Geometry check sheet. Reference: the model listing, model coordinates, mm. A direction names the side the tool comes from. Give positions to 0.01 mm unless a question says otherwise; leave off trailing zeros. Write each loop counter-clockwise with the first axis right and the second up, starting at its lowest first coordinate (ties: lowest second). Pieces come first, ordered by that corner, then holes. Notation, with made-up numbers: (-15, 15) -> (6, 15) arc R32 cw to (6, 49) -> close; hole circle Ø5 at (75, -20). An arc over 180 degrees is marked (long way). Use a Markdown table: item, result. Add a question column.
Autodesk Inventor part; units mm, degrees
ref_plane "YZ Plane" through (0, 0, 0) normal (1, 0, 0) x (0, 1, 0)
ref_plane "XZ Plane" through (0, 0, 0) normal (0, 1, 0) x (-1, 0, 0)
ref_plane "XY Plane" through (0, 0, 0) normal (0, 0, 1) x (1, 0, 0)
sketch "Эскиз1" plane through (0, 0, 0) normal (0, 1, 0) x (-1, 0, 0)
  line L0 (-155, 270) -> (155, 270)
  line L1 (155, 270) -> (155, -270)
  line L2 (155, -270) -> (-155, -270)
  line L3 (-155, -270) -> (-155, 270)
  line L4 (-155, 270) -> (155, -270) construction
  line L5 (155, 270) -> (-155, -270) construction
  circle A0 centre (0, 0) radius 50
  dimension "d0" = 310
  dimension "d1" = 540
  dimension "d2" = 100
extrude "Выдавливание1" add sketch "Эскиз1" along normal blind 4
sketch "Эскиз2" plane through (0, 4, 0) normal (0, 1, 0) x (1, 0, 0)
  line L0 (153, 268) -> (-153, 268)
  line L1 (-153, 268) -> (-153, -268)
  line L2 (-153, -268) -> (153, -268)
  line L3 (153, -268) -> (153, 268)
  line L4 (153, 268) -> (-153, -268) construction
  line L5 (-153, 268) -> (153, -268) construction
  line L6 (-155, 270) -> (-155, -270)
  line L7 (155, 270) -> (-155, 270)
  line L8 (-155, 270) -> (-155, -270)
  line L9 (-155, -270) -> (155, -270)
  line L10 (155, -270) -> (155, 270)
  line L11 (155, 270) -> (-155, -270) construction
  line L12 (-155, 270) -> (155, -270) construction
  point P0 (0, 0)
  dimension "d5" = 306
  dimension "d6" = 536
extrude "Выдавливание2" add sketch "Эскиз2" along normal blind 40
sketch "Эскиз3" plane through (0, 4, 0) normal (0, 1, 0) x (1, 0, 0)
  circle A0 centre (0, 0) radius 50
  circle A1 centre (0, 0) radius 60
  dimension "d9" = 120
extrude "Выдавливание3" add sketch "Эскиз3" along normal blind 40
properties part number "ЗЕМЛЯЕМКОСТЬ"
1) Sectioned sample at D-D, the plane x = -110. Enter the section's corners in (y, z), and give its area (3 significant figures).
2) Sectioned sample at B-B, the plane z = 0. Enter the section's corners in (x, y), and give its area (3 significant figures).
3) Material ranges on probe 1 along Z at (x, y) = (0, 31); probe 2 along X at (y, z) = (23.5, 0); probe 3 along X at (y, z) = (35, -207), recorded low to high. Write a range as [from, to].
4) Gauge pin test, flat end, axial feed: P1, Ø5, axis at x = 55, z = 112, coming from the +Y side. Record the tip position at first contact, or that the pin passes through.
5) Sectioned sample at A-A, the plane y = 14. Enter the section's corners in (x, z), and give its area (3 significant figures).
6) Tool access check on faces 1 (the face through (-2, 22, -270)), 2 (the face through (-2, 24, 268)). Record the directions out of +Z, -Z, +X, -X, +Y, -Y that give a thin tool (end or side, any length) a straight path to the whole face; none if there is none.
7) Draft check along X on faces 3 (the face through (-155, 22, 4)), 4 (the face through (-23, 44, -45)), 5 (the face through (-153, 24, -4)). Enter one of: +X half, -X half, draft (parallel to the pull), parting line (faces both ways), or undercut.
8) Sectioned sample at C-C, the plane x = 0. Enter the section's corners in (y, z).
Check values:
| question | item | result |
|---|---|---|
| 1 | outline | (0, -270) -> (44, -270) -> (44, -268) -> (4, -268) -> (4, 268) -> (44, 268) -> (44, 270) -> (0, 270) -> close |
| 1 | area | 2,320 mm² |
| 2 | outline | (-155, 0) -> (-50, 0) -> (-50, 44) -> (-60, 44) -> (-60, 4) -> (-153, 4) -> (-153, 44) -> (-155, 44) -> close; (50, 0) -> (155, 0) -> (155, 44) -> (153, 44) -> (153, 4) -> (60, 4) -> (60, 44) -> (50, 44) -> close |
| 2 | area | 1,800 mm² |
| 3 | probe 1 | [-270, -268], [-60, -50], [50, 60], [268, 270] |
| 3 | probe 2 | [-155, -153], [-60, -50], [50, 60], [153, 155] |
| 3 | probe 3 | [-155, -153], [153, 155] |
| 4 | P1 | y = 4 |
| 5 | outline | (-155, -270) -> (155, -270) -> (155, 270) -> (-155, 270) -> close; circle Ø120 at (0, 0); hole (-153, -268) -> (153, -268) -> (153, 268) -> (-153, 268) -> close; hole circle Ø100 at (0, 0) |
| 5 | area | 6,840 mm² |
| 6 | face 1 | -Z, +X, -X, +Y, -Y |
| 6 | face 2 | +Y |
| 7 | face 3 | -X half |
| 7 | face 4 | draft |
| 7 | face 5 | undercut |
| 8 | outline | (0, -270) -> (44, -270) -> (44, -268) -> (4, -268) -> (4, -60) -> (44, -60) -> (44, -50) -> (0, -50) -> close; (0, 50) -> (44, 50) -> (44, 60) -> (4, 60) -> (4, 268) -> (44, 268) -> (44, 270) -> (0, 270) -> close |
